The drawing under review shows one solid part. Ordinate dimensions are in mm from its lowest x, y, z. Round coordinates to 2 decimals unless told otherwise and drop trailing zeros. Write each loop counter-clockwise with the first axis right and the second up, starting at its lowest first coordinate (ties: lowest second). Pieces come first, ordered by that corner, then holes. Notation, with made-up numbers: (57.25, -11) -> (70.25, -11) arc R21 cw to (70.25, 15) -> close; hole circle Ø9 at (41, -38.75). An arc over 180 degrees is marked (long way). Write item = value, one per line. Start each with the question number.
Item 1: Add section B-B, the plane z = 40. State the section outline as (x, y) points.
Item 2: To check wall thickness, follow L1, parallel to X at y = 0.2, z = 38. State the ranges of the line that lie inside material, in increasing order.
Item 3: Add section A-A, the plane y = 1.2. State the section outline as (x, z) points, then the cut area to 3 significant figures.
Item 4: For pin 1 Ø0.6 at (y, z) = (0.5, 7.5) entering from -X; pin 2 Ø0.6 at (x, y) = (1, 1) entering from -Z; pin 3 Ø1 at (y, z) = (1, 10) entering from +X, all flat-tipped, find the tip position at first contact; note any pin that passes through.
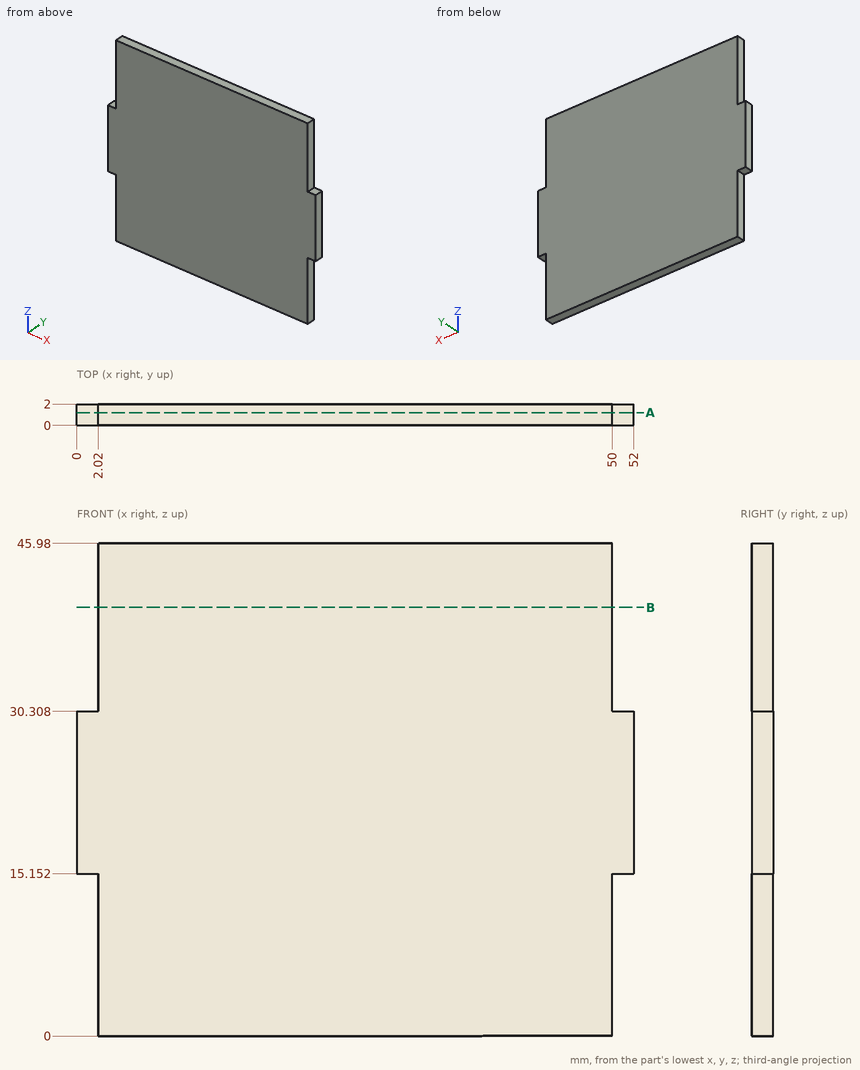
Result set:
q1.outline = (2.02, 0) -> (50, 0) -> (50, 2) -> (2.02, 2) -> close
q2.L1 = 2.02 to 50
q3.outline = (0, 15.15) -> (2.02, 15.15) -> (2.02, 0) -> (50, 0) -> (50, 15.15) -> (52, 15.15) -> (52, 30.31) -> (50, 30.31) -> (50, 45.98) -> (2.02, 45.98) -> (2.02, 30.31) -> (0, 30.31) -> close
q3.area = 2,270 mm²
q4.pin_1 = 2.02
q4.pin_2 = 15.15
q4.pin_3 = 50
